```python
from build123d import *

# Parameters (mm, degrees)
SKETCH1_R           = 1.5
BOSS_EXTRUDE1_DEPTH = 16
SKETCH2_R           = 2.8
BOSS_EXTRUDE2_DEPTH = 2.4
FILLET1_R           = 1
CUT_EXTRUDE1_DEPTH  = 1
CHAMFER1_SIZE       = 0.5


with BuildPart() as part:
    # Sketch1 → Boss-Extrude1 (new body)
    with BuildSketch(Plane(origin=(0, 0, 0), x_dir=(1, 0, 0), z_dir=(0, 1, 0))):
        with Locations(Location((0, 0, 0), (0, 0, 270))):
            Circle(SKETCH1_R)
    extrude(amount=BOSS_EXTRUDE1_DEPTH)

    # Sketch2 → Boss-Extrude2 (add)
    with BuildSketch(Plane(origin=(0, 16, 0), x_dir=(1, 0, 0), z_dir=(0, 1, 0))):
        with Locations(Location((0, 0, 0), (0, 0, 270))):
            Circle(SKETCH2_R)
    extrude(amount=BOSS_EXTRUDE2_DEPTH)

    # Fillet1
    fillet1_edges = [part.edges().sort_by_distance(p)[0] for p in [
        (0, 18.4, -2.8),
    ]]
    fillet(fillet1_edges, radius=FILLET1_R)

    # Sketch3 → Cut-Extrude1 (cut)
    with BuildSketch(Plane(origin=(0, 18.4, 0), x_dir=(1, 0, 0), z_dir=(0, 1, 0))):
        Polygon((1.8, 0), (0.9, 1.558845727), (-0.9, 1.558845727), (-1.8, 0), (-0.9, -1.558845727), (0.9, -1.558845727), align=None)
    extrude(amount=-CUT_EXTRUDE1_DEPTH, mode=Mode.SUBTRACT)

    # Chamfer1
    chamfer1_edges = [part.edges().sort_by_distance(p)[0] for p in [
        (0, 0, -1.5),
    ]]
    chamfer(chamfer1_edges, length=CHAMFER1_SIZE)


solid = part.part
```
CAD build for the part. Positions are in the model's coordinates, mm. A direction names the side the tool comes from. Round coordinates to 2 decimals unless told otherwise and drop trailing zeros. Order: outer loops, then holes, each group sorted by start corner. A loop starts at its lowest first (then second) coordinate and runs counter-clockwise, first axis right, second up. Notation, with made-up numbers: (-23.75, -25) -> (12.25, -25) arc R11 cw to (12.25, -8) -> close; hole circle Ø6 at (24.25, -10.75). An arc over 180 degrees is marked (long way). Write item = value, one per line.
(1) 3-axis set-ups, long thin cutter, end or side, ignore diameter. For faces 4 (the flat face through (0, 0, 0)), 5 (the flat face through (0, 17.4, 0)): which of +Z, -Z, +X, -X, +Y, -Y reach the whole face in a straight line?
Answers follow:
face_4 = +Z, -Z, +X, -X, -Y
face_5 = +Y
(2) Cut at B-B (y = 17). Write the cut outline in (x, z), plus the area to 3 significant figures.
Answers follow:
outline = circle Ø5.6 at (0, 0)
area = 24.6 mm²
(3) Cut at A-A (x = 0). Write the cut outline in (y, z).
Answers follow:
outline = (0, -1) -> (0.5, -1.5) -> (16, -1.5) -> (16, -2.8) -> (17.4, -2.8) arc R1 ccw to (18.4, -1.8) -> (18.4, -1.56) -> (17.4, -1.56) -> (17.4, 1.56) -> (18.4, 1.56) -> (18.4, 1.8) arc R1 ccw to (17.4, 2.8) -> (16, 2.8) -> (16, 1.5) -> (0.5, 1.5) -> (0, 1) -> close
(4) Drill centre lines: L1, parallel to Y at x = 0.05, z = 1.75; L2, parallel to Y at x = 0.6, z = 0.3; L3, parallel to X at y = 11.5, z = 1.2. Where is each one in solid material? Low to high.
Answers follow:
L1 = 16 to 18.4
L2 = 0 to 17.4
L3 = -0.9 to 0.9
(5) Flat gauge pins, fed straight in: P1, Ø0.9, axis at x = 0, z = 0, coming from the +Y side; P2, Ø0.8, axis at x = 0, y = 18, coming from the +Z side; P3, Ø1.5, axis at y = 14, z = -2, coming from the +X side. Where does each tip first touch, or does it go through?
Answers follow:
P1 = 17.4
P2 = 2.78
P3 = 0.83
(6) Pull direction Z, two halves, no side cores. Call faces 1 (the cylindrical face through (0.45, 8.14, 1.43)), 2 (the flat face through (1.356, 17.907, -0.769)), 3 (the flat face through (-1.2, 16, 1.2)): +Z half, -Z half, draft (parallel to the pull), parting line (faces both ways), or undercut.
Answers follow:
face_1 = parting line
face_2 = undercut
face_3 = draft
